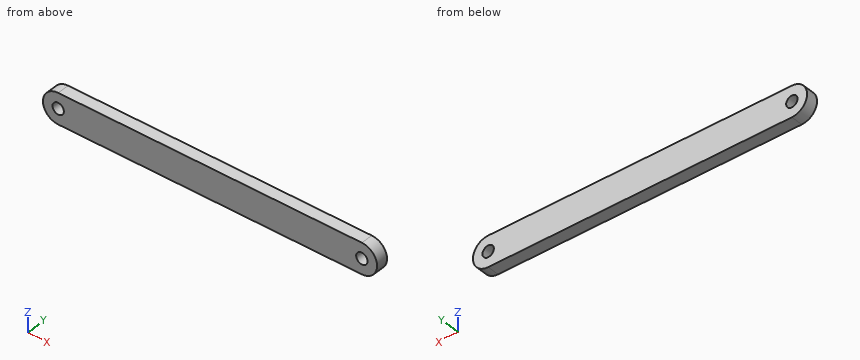
from build123d import *

# Parameters (mm, degrees)
SKETCH1_R           = 1.497293459
BOSS_EXTRUDE1_DEPTH = 3.175


with BuildPart() as part:
    # Sketch1 → Boss-Extrude1 (new body)
    with BuildSketch(Plane(origin=(0, 0, 0), x_dir=(1, 0, 0), z_dir=(0, 1, 0))):
        with BuildLine():
            Line((40.018335965, 4.000091093), (-39.839960243, 4.000091093))
            ThreePointArc((-39.839960243, 4.000091093), (-43.840051334, 2e-09), (-39.839960243, -4.000091089))
            Line((-39.839960243, -4.000091089), (40.018335965, -4.000091089))
            ThreePointArc((40.018335965, -4.000091089), (44.018427056, 2e-09), (40.018335965, 4.000091093))
        make_face()
        with Locations(Location((-39.839960243, 2e-09, 0), (0, 0, 270))):
            Circle(SKETCH1_R, mode=Mode.SUBTRACT)
        with Locations(Location((40.018335965, 2e-09, 0), (0, 0, 270))):
            Circle(SKETCH1_R, mode=Mode.SUBTRACT)
    extrude(amount=BOSS_EXTRUDE1_DEPTH)


solid = part.part
The listing builds one solid part. Answer for the finished solid, in the listing's coordinates (mm). Round coordinates to 2 decimals unless told otherwise and drop trailing zeros. Write each loop counter-clockwise with the first axis right and the second up, starting at its lowest first coordinate (ties: lowest second). Pieces come first, ordered by that corner, then holes. Notation, with made-up numbers: (76, 33.5) - (86, 33.5) arc R32 cw to (86, 59.5) - close; hole circle Ø11 at (27, 25). An arc over 180 degrees is marked (long way). Use a Markdown table: item, result. Add a question column.
1. The part is cut by section A-A (z = 0). Write down the section's boundary in (x, y) (3 decimals), and give its area (3 significant figures).
2. The part is cut by section C-C (z = 3.25). Write down the section's boundary in (x, y) (3 decimals), and give its area (3 significant figures).
3. The part is cut by section B-B (y = 1.8). Write down the section's boundary in (x, z), and give its area (3 significant figures).
4. Consider line 1 (X direction, y = 1.15, z = 0); line 2 (X direction, y = 1.8, z = -1.25); line 3 (Z direction, x = -40, y = 3). Determine where each line is inside the solid, lowest interval first.
Reported:
| question | item | result |
|---|---|---|
| 1 | outline | (-43.84, 0) - (-41.337, 0) - (-41.337, 3.175) - (-43.84, 3.175) - close; (-38.343, 0) - (38.521, 0) - (38.521, 3.175) - (-38.343, 3.175) - close; (41.516, 0) - (44.018, 0) - (44.018, 3.175) - (41.516, 3.175) - close |
| 1 | area | 260 mm^2 |
| 2 | outline | (-42.172, 0) - (42.35, 0) - (42.35, 3.175) - (-42.172, 3.175) - close |
| 2 | area | 268 mm^2 |
| 3 | outline | (-39.84, -4) - (40.02, -4) arc R4 ccw to (40.02, 4) - (-39.84, 4) arc R4 ccw to start; hole circle Ø2.99 at (-39.84, 0); hole circle Ø2.99 at (40.02, 0) |
| 3 | area | 675 mm^2 |
| 4 | line 1 | -43.84 to -41.34, -38.34 to 38.52, 41.52 to 44.02 |
| 4 | line 2 | -43.64 to -40.66, -39.02 to 39.19, 40.84 to 43.82 |
| 4 | line 3 | -4 to -1.49, 1.49 to 4 |
